from build123d import *

# Parameters (mm, degrees)
SKETCH_W     = 15
SKETCH_H     = 95
PAD_DEPTH    = 2
PAD001_DEPTH = 1.5


with BuildPart() as part:
    # Sketch → Pad (new body)
    with BuildSketch(Plane.XY):
        Rectangle(SKETCH_W, SKETCH_H)
    extrude(amount=PAD_DEPTH)

    # Sketch001 (on DatumPlane) → Pad001 (join, symmetric)
    with BuildSketch(Plane(origin=(0, 27.5, 0), x_dir=(-1, 0, 0), z_dir=(0, 1, 0))):
        Polygon((-4, 2), (-4, 10.5), (-2, 10.5), (-1, 9.5), (-2, 8.5), (-2, 2), align=None)
        Polygon((4, 2), (4, 10.5), (2, 10.5), (1, 9.5), (2, 8.5), (2, 2), align=None)
    pad001 = extrude(amount=PAD001_DEPTH, both=True)

    # Mirrored: Pad001 across XZ
    add(pad001.mirror(Plane.XZ))


solid = part.part
The model under review builds one solid part; all positions refer to its coordinate system, in mm. A direction names the side the tool comes from. Give positions to 0.01 mm unless a question says otherwise; leave off trailing zeros. Write each loop counter-clockwise with the first axis right and the second up, starting at its lowest first coordinate (ties: lowest second). Pieces come first, ordered by that corner, then holes. Notation, with made-up numbers: M -22,27 L 2,27 A25 ccw 2,55 Z; hole C 44.5,46.25 d2. An arc over 180 degrees is marked long. One line per question, with ' | ' between items. Start each with the question number.
Item 1: For faces 4 (the flat face through (2, -27, 5)), 5 (the flat face through (3, -26, 6)), 6 (the flat face through (3, -29, 6)), 7 (the flat face through (-3, 29, 6)), list the 3-axis set-ups (+Z, -Z, +X, -X, +Y, -Y) from which the entire face can be reached by the end or side of a thin tool; tool diameter is ignored.
Item 2: We need section C-C on y = 13. Write out the cut boundary in (x, z), plus the area to 3 significant figures.
Item 3: For pin 1 (2.5 mm diameter, centred on y = 27, z = 5, fed in from -X); pin 2 (2.5 mm diameter, centred on y = 27.5, z = 5.5, fed in from +X); pin 3 (3.5 mm diameter, centred on x = 3, z = 5, fed in from +Y), all flat-tipped, find the tip position at first contact; note any pin that passes through.
Item 4: We need section A-A on z = 5.25. Write out the cut boundary in (x, y), plus the area to 3 significant figures.
Item 5: Draft analysis for pull direction X (two halves, no side actions). For faces 1 (the flat face through (3, -27, 10.5)), 2 (the flat face through (-2, -28, 5)), 3 (the flat face through (-7.5, -1, 1)), state which applies: released by +X, released by -X, zero draft, split by the parting line, or undercut.
Item 6: Wall thickness on line 1 (Y direction, x = -2.25, z = 6.25); line 2 (X direction, y = -27.5, z = 5); line 3 (Z direction, x = 0, y = 24.5): over which ranges is each line inside the solid? List them lowest first. Write a range as from..to.
Item 7: We need section B-B on x = 5.25. Write out the cut boundary in (y, z).
Results found:
1) face 4: +Y, -Y | face 5: +Z, +X, -X | face 6: +Z, +X, -X, -Y | face 7: +Z, +X, -X, +Y
2) outline: M -7.5,0 L 7.5,0 L 7.5,2 L -7.5,2 Z | area: 30.0 mm2
3) pin 1: stops at x = -4 | pin 2: stops at x = 4 | pin 3: stops at y = 29
4) outline: M -4,-29 L -2,-29 L -2,-26 L -4,-26 Z; M -4,26 L -2,26 L -2,29 L -4,29 Z; M 2,-29 L 4,-29 L 4,-26 L 2,-26 Z; M 2,26 L 4,26 L 4,29 L 2,29 Z | area: 24.0 mm2
5) face 1: zero draft | face 2: undercut | face 3: released by -X
6) line 1: y = -29..-26, 26..29 | line 2: x = -4..-2, 2..4 | line 3: z = 0..2
7) outline: M -47.5,0 L 47.5,0 L 47.5,2 L -47.5,2 Z
